Can you work these out from the drawing? Everything is in mm from the part's minimum corner. A direction names the side the tool comes from. Coordinates: 2 decimals unless noted, no trailing zeros. Write each loop counter-clockwise with the first axis right and the second up, starting at its lowest first coordinate (ties: lowest second). Pieces come first, ordered by that corner, then holes.
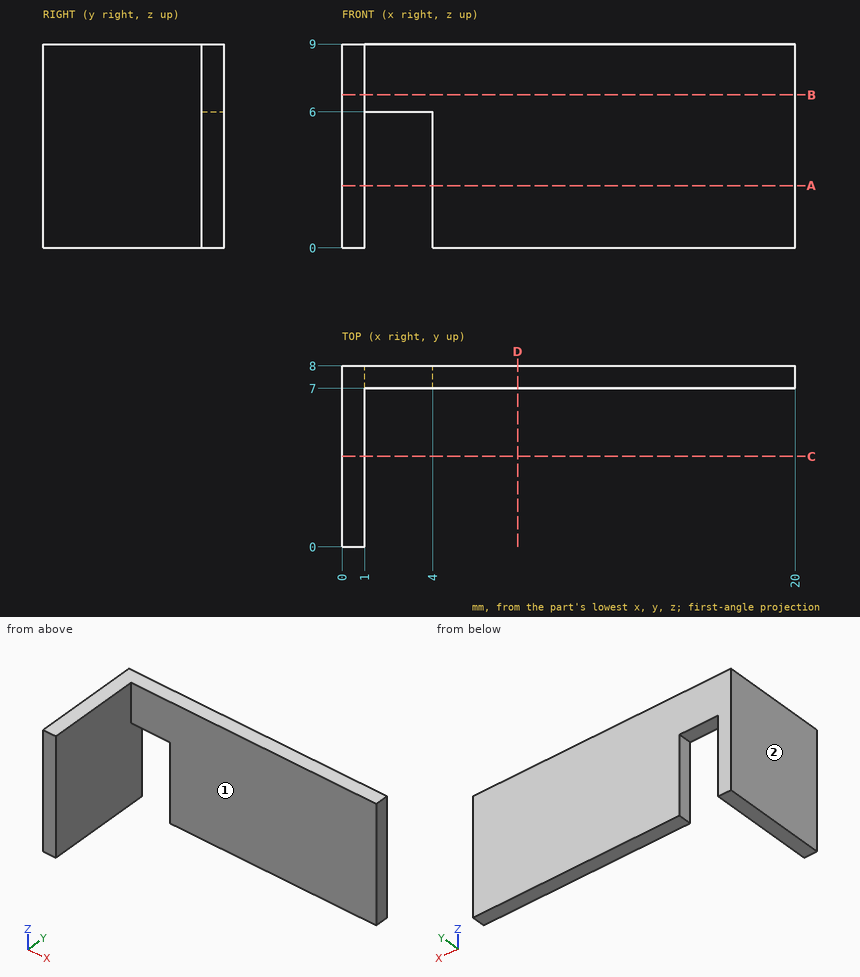
1. If I drill on line 1 (Y direction, x = 2.25, z = 8.25); line 2 (X direction, y = 4.75, z = 1.5), over which ranges is the centre line in solid material (lowest first)?
2. I want a section at C-C (y = 4). List the corners of the cut face in (x, z) for me, then the cut area to 3 significant figures.
3. I want a section at A-A (z = 2.75). List the corners of the cut face in (x, y) for me, then the cut area to 3 significant figures.
4. I want a section at B-B (z = 6.75). List the corners of the cut face in (x, y) for me, then the cut area to 3 significant figures.
5. On a 3-axis mill with a long thin cutter (end or side, diameter ignored), from which of +Z, -Z, +X, -X, +Y, -Y can I reach the whole of each face in a straight line? I mean the marked faces 1 and 2. Say none if no direction works.
6. For pin 1 Ø2.5 at (y, z) = (2.5, 5) entering from +X; pin 2 Ø3 at (x, z) = (17, 8) entering from -Y; pin 3 Ø1.1 at (x, y) = (2, 7.5) entering from -Z, each with a flat end and sliding along its axis, tell me the tip position at first contact or that it passes through.
7. I want a section at D-D (x = 7.75). List the corners of the cut face in (y, z) for me.
Response values:
1. line 1: y = 7 to 8
1. line 2: x = 0 to 1
2. outline: (0, 0) - (1, 0) - (1, 9) - (0, 9) - close
2. area: 9.00 mm2
3. outline: (0, 0) - (1, 0) - (1, 8) - (0, 8) - close; (4, 7) - (20, 7) - (20, 8) - (4, 8) - close
3. area: 24.0 mm2
4. outline: (0, 0) - (1, 0) - (1, 7) - (20, 7) - (20, 8) - (0, 8) - close
4. area: 27.0 mm2
5. face 1: +Z, -Z, +X, -Y
5. face 2: +Z, -Z, -X, +Y, -Y
6. pin 1: stops at x = 1
6. pin 2: stops at y = 7
6. pin 3: stops at z = 6
7. outline: (7, 0) - (8, 0) - (8, 9) - (7, 9) - close
